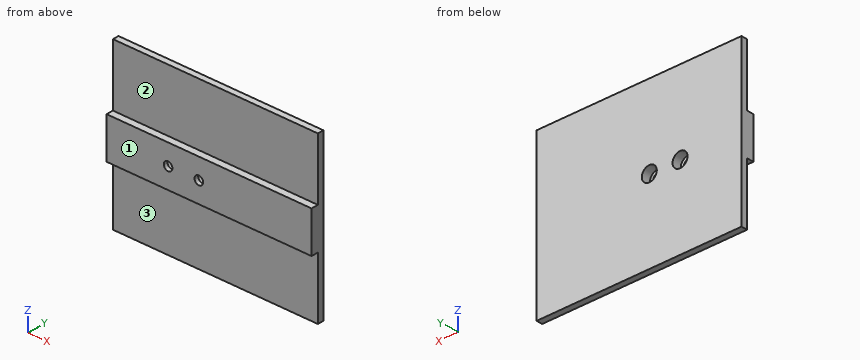
from build123d import *

# Parameters (mm, degrees)
SKETCH_1_W                   = 100
SKETCH_1_H                   = 80
EXTRUDE_1_DEPTH              = 3
SKETCH_2_W                   = 100
SKETCH_2_H                   = 20
EXTRUDE_2_DEPTH              = 3.4
HOLE_WIZARD_M4_1_D           = 4.2
HOLE_WIZARD_M4_1_CBORE_D     = 7.3
HOLE_WIZARD_M4_1_CBORE_DEPTH = 4.4


with BuildPart() as part:
    # 草圖1 → 填料-伸長1 (new body)
    with BuildSketch(Plane(origin=(0, 0, 0), x_dir=(1, 0, 0), z_dir=(0, 1, 0))):
        Rectangle(SKETCH_1_W, SKETCH_1_H)
    extrude(amount=EXTRUDE_1_DEPTH)

    # 草圖2 → 填料-伸長2 (add)
    with BuildSketch(Plane.XZ):
        Rectangle(SKETCH_2_W, SKETCH_2_H)
    extrude(amount=EXTRUDE_2_DEPTH)

    # M4 六角承窩頭蓋螺釘的柱孔1 (through all)
    with Locations(Plane(origin=(0, 3, 0), x_dir=(1, 0, 0), z_dir=(0, 1, 0))):
        with Locations((-20, 0), (-5, 0)):
            CounterBoreHole(HOLE_WIZARD_M4_1_D / 2, HOLE_WIZARD_M4_1_CBORE_D / 2, HOLE_WIZARD_M4_1_CBORE_DEPTH)


solid = part.part
Design review of the part built by this model. Coordinates are the model's own, in mm. Face numbers are marked on the shaded views. A direction names the side the tool comes from. Coordinates: 2 decimals unless noted, no trailing zeros. Loops run counter-clockwise (first coordinate to the right, second up) from the corner with the lowest first, then second, coordinate; pieces in that order, holes last.
Item 1: Add section C-C (x = 25). Write out the cut boundary in (y, z), and give its area (3 significant figures).
Completed:
outline: (-3.4, -10) - (0, -10) - (0, -40) - (3, -40) - (3, 40) - (0, 40) - (0, 10) - (-3.4, 10) - close
area: 308 mm2
Item 2: For the marked faces 1, 2 and 3, list the 3-axis set-ups (+Z, -Z, +X, -X, +Y, -Y) from which the entire face can be reached by the end or side of a thin tool; tool diameter is ignored.
Completed:
face 1: +Z, -Z, +X, -X, -Y
face 2: +Z, +X, -X, -Y
face 3: -Z, +X, -X, -Y
Item 3: Add section B-B (x = -20). Write out the cut boundary in (y, z).
Completed:
outline: (-3.4, -10) - (0, -10) - (0, -40) - (3, -40) - (3, -3.65) - (-1.4, -3.65) - (-1.4, -2.1) - (-3.4, -2.1) - close; (-3.4, 2.1) - (-1.4, 2.1) - (-1.4, 3.65) - (3, 3.65) - (3, 40) - (0, 40) - (0, 10) - (-3.4, 10) - close
Item 4: Add section A-A (z = 0). Write out the cut boundary in (x, y), and give its area (3 significant figures).
Completed:
outline: (-50, -3.4) - (-22.1, -3.4) - (-22.1, -1.4) - (-23.65, -1.4) - (-23.65, 3) - (-50, 3) - close; (-17.9, -3.4) - (-7.1, -3.4) - (-7.1, -1.4) - (-8.65, -1.4) - (-8.65, 3) - (-16.35, 3) - (-16.35, -1.4) - (-17.9, -1.4) - close; (-2.9, -3.4) - (50, -3.4) - (50, 3) - (-1.35, 3) - (-1.35, -1.4) - (-2.9, -1.4) - close
area: 559 mm2
Item 5: Add section D-D (z = -18). Write out the cut boundary in (x, y), and give its area (3 significant figures).
Completed:
outline: (-50, 0) - (50, 0) - (50, 3) - (-50, 3) - close
area: 300 mm2
Item 6: Wall thickness on L1, parallel to Z at x = -20, y = -0.05; L2, parallel to Z at x = -20, y = -2.5; L3, parallel to X at y = -1, z = 3: over which ranges is each line inside the solid? List them lowest first.
Completed:
L1: z = -10 to -3.65, 3.65 to 10
L2: z = -10 to -2.1, 2.1 to 10
L3: x = -50 to -22.08, -17.92 to -7.08, -2.92 to 50
Item 7: Clearance check with flat-ended pins moving along their axes: pin 1 (2 mm diameter, centred on x = -19, z = 1.5, fed in from +Y); pin 2 (1 mm diameter, centred on x = -10.5, y = -2, fed in from +Z); pin 3 (3 mm diameter, centred on x = -9, z = -19.5, fed in from -Y); pin 4 (4 mm diameter, centred on x = -20, z = 0, fed in from -Y). State where each tip first meets the part, or that it passes through.
Completed:
pin 1: stops at y = -1.4
pin 2: stops at z = 10
pin 3: stops at y = 0
pin 4: passes through
